The listing builds one solid part. Answer for the finished solid, in the listing's coordinates (mm). A direction names the side the tool comes from. Give positions to 0.01 mm unless a question says otherwise; leave off trailing zeros. Write each loop counter-clockwise with the first axis right and the second up, starting at its lowest first coordinate (ties: lowest second). Pieces come first, ordered by that corner, then holes. Notation, with made-up numbers: (24.5, 85) -> (32.5, 85) arc R30 ccw to (32.5, 119) -> close; hole circle Ø11 at (49, 0). An arc over 180 degrees is marked (long way). Put each result on its own line as item: value. Start each with the question number.
1) A cutting plane is placed at C-C (y = -26.5). Write down the section's boundary in (x, z), then the cut area to 3 significant figures.
2) Flat-ended cylindrical pins translate along their axes: pin 1 Ø1 at (y, z) = (-30, -13.5) entering from -X; pin 2 Ø8 at (x, y) = (2.5, -33.5) entering from -Z; pin 3 Ø1.5 at (x, y) = (16.5, -15.5) entering from -Z; pin 4 Ø5.5 at (x, z) = (0, 0) entering from -Y. Find the tip coordinate at first contact, or state that the pin passes through.
3) For a pull along X with two mould halves and no side action, classify faces 1 (the conical face through (31.82, -14.81, -7.07)), 2 (the flat face through (-17, -2, -14)), 3 (the flat face through (0, 0, -6)) as released by +X, released by -X, zero draft, split by the parting line, or undercut.
4) A cutting plane is placed at B-B (y = -8). Give the number of separate pieces and of enclosed holes in the cut face, then the cut area to 3 significant figures.
5) Find the intervals of material crossed by line 1 along X through (y, z) = (-6, 0); line 2 along X through (y, z) = (-3.5, 0); line 3 along X through (y, z) = (-41, -33.5), in increasing order. Write a range as from..to.
6) For faces 4 (the cylindrical face through (14.087, -52.986, -44.734)), 5 (the flat face through (14, -2, 17)), 6 (the cylindrical face through (9.36, -11.52, -5.97)), determine the directions among +Z, -Z, +X, -X, +Y, -Y from which every point of the face is accessible in a straight line to the end or side of a thin tool.
7) A cutting plane is placed at A-A (y = -34). Write down the section's boundary in (x, z), then the cut area to 3 significant figures.
from build123d import *

# Parameters (mm, degrees)
SKETCH_2_R          = 1.75
CUT_EXTRUDE_1_DEPTH = 85.280602751
CUT_EXTRUDE_2_DEPTH = 8
SKETCH_4_R          = 3
CUT_EXTRUDE_3_DEPTH = 2
SKETCH_5_R          = 11.1
CUT_EXTRUDE_4_DEPTH = 2.2
SKETCH_6_R          = 4.5
CUT_EXTRUDE_5_DEPTH = 79.292911557
SKETCH_7_R          = 46.9
SKETCH_7_R_2        = 40
EXTRUDE_1_DEPTH     = 2


with BuildPart() as part:
    # 草图1 → 旋转1 (revolve)
    with BuildSketch(Plane.XY, mode=Mode.PRIVATE) as revolve_1_sk:
        Polygon((0, 0), (26.9, 0), (46.9, -52), (43.553846154, -52), (28.4, -12.6), (26.9, -12.6), (0, -12.6), align=None)
    revolve(revolve_1_sk.sketch.rotate(Axis((0, 0, 0), (0, -1, 0)), 90), axis=Axis((0, 0, 0), (0, -1, 0)))

    # 草图2 → 切除-拉伸1 (cut, through all)
    with BuildSketch(Plane(origin=(0, 0, 0), x_dir=(1, 0, 0), z_dir=(0, 1, 0))):
        with BuildLine():
            Line((-15.5, 13.75), (-15.5, 15.5))
            Line((-15.5, 15.5), (-13.75, 15.5))
            ThreePointArc((-13.75, 15.5), (-16.737436867, 16.737436867), (-15.5, 13.75))
        make_face()
        with BuildLine():
            Line((-13.75, 15.5), (-15.5, 15.5))
            Line((-15.5, 15.5), (-15.5, 13.75))
            ThreePointArc((-15.5, 13.75), (-14.262563133, 14.262563133), (-13.75, 15.5))
        make_face()
        with BuildLine():
            Line((-15.5, 13.75), (-15.5, 15.5))
            Line((-15.5, 15.5), (-13.75, 15.5))
            ThreePointArc((-13.75, 15.5), (-16.737436867, 16.737436867), (-15.5, 13.75))
        make_face()
        with BuildLine():
            Line((-13.75, 15.5), (-15.5, 15.5))
            Line((-15.5, 15.5), (-15.5, 13.75))
            ThreePointArc((-15.5, 13.75), (-14.262563133, 14.262563133), (-13.75, 15.5))
        make_face()
        with BuildLine():
            ThreePointArc((17.25, 15.5), (15.5, 17.25), (13.75, 15.5))
            Line((13.75, 15.5), (15.5, 15.5))
            Line((15.5, 15.5), (15.5, 13.75))
            ThreePointArc((15.5, 13.75), (16.737436867, 14.262563133), (17.25, 15.5))
        make_face()
        with BuildLine():
            Line((15.5, 15.5), (13.75, 15.5))
            ThreePointArc((13.75, 15.5), (14.262563133, 14.262563133), (15.5, 13.75))
            Line((15.5, 13.75), (15.5, 15.5))
        make_face()
        with BuildLine():
            ThreePointArc((17.25, 15.5), (15.5, 17.25), (13.75, 15.5))
            Line((13.75, 15.5), (15.5, 15.5))
            Line((15.5, 15.5), (15.5, 13.75))
            ThreePointArc((15.5, 13.75), (16.737436867, 14.262563133), (17.25, 15.5))
        make_face()
        with BuildLine():
            Line((15.5, 15.5), (13.75, 15.5))
            ThreePointArc((13.75, 15.5), (14.262563133, 14.262563133), (15.5, 13.75))
            Line((15.5, 13.75), (15.5, 15.5))
        make_face()
        with BuildLine():
            ThreePointArc((17.25, -15.5), (16.737436867, -14.262563133), (15.5, -13.75))
            Line((15.5, -13.75), (15.5, -15.5))
            Line((15.5, -15.5), (13.75, -15.5))
            ThreePointArc((13.75, -15.5), (15.5, -17.25), (17.25, -15.5))
        make_face()
        with BuildLine():
            Line((15.5, -15.5), (15.5, -13.75))
            ThreePointArc((15.5, -13.75), (14.262563133, -14.262563133), (13.75, -15.5))
            Line((13.75, -15.5), (15.5, -15.5))
        make_face()
        with BuildLine():
            ThreePointArc((17.25, -15.5), (16.737436867, -14.262563133), (15.5, -13.75))
            Line((15.5, -13.75), (15.5, -15.5))
            Line((15.5, -15.5), (13.75, -15.5))
            ThreePointArc((13.75, -15.5), (15.5, -17.25), (17.25, -15.5))
        make_face()
        with BuildLine():
            Line((15.5, -15.5), (15.5, -13.75))
            ThreePointArc((15.5, -13.75), (14.262563133, -14.262563133), (13.75, -15.5))
            Line((13.75, -15.5), (15.5, -15.5))
        make_face()
        with BuildLine():
            ThreePointArc((-13.75, -15.5), (-14.262563133, -14.262563133), (-15.5, -13.75))
            Line((-15.5, -13.75), (-15.5, -15.5))
            Line((-15.5, -15.5), (-13.75, -15.5))
        make_face()
        with BuildLine():
            Line((-15.5, -15.5), (-15.5, -13.75))
            ThreePointArc((-15.5, -13.75), (-16.737436867, -16.737436867), (-13.75, -15.5))
            Line((-13.75, -15.5), (-15.5, -15.5))
        make_face()
        with BuildLine():
            ThreePointArc((-13.75, -15.5), (-14.262563133, -14.262563133), (-15.5, -13.75))
            Line((-15.5, -13.75), (-15.5, -15.5))
            Line((-15.5, -15.5), (-13.75, -15.5))
        make_face()
        with BuildLine():
            Line((-15.5, -15.5), (-15.5, -13.75))
            ThreePointArc((-15.5, -13.75), (-16.737436867, -16.737436867), (-13.75, -15.5))
            Line((-13.75, -15.5), (-15.5, -15.5))
        make_face()
        with Locations(Location((0, 21.920310217, 0), (0, 0, 270))):
            Circle(SKETCH_2_R)
        with Locations(Location((-21.920310217, 0, 0), (0, 0, 270))):
            Circle(SKETCH_2_R)
        with Locations(Location((21.920310217, 0, 0), (0, 0, 270))):
            Circle(SKETCH_2_R)
        with Locations(Location((0, -21.920310217, 0), (0, 0, 270))):
            Circle(SKETCH_2_R)
    extrude(amount=-CUT_EXTRUDE_1_DEPTH, mode=Mode.SUBTRACT)

    # 草图3 → 切除-拉伸2 (cut)
    with BuildSketch(Plane.XZ.offset(12.6)):
        Polygon((2.086344802, -19.833965415), (0, -21.920310217), (-2.086344802, -19.833965415), (-3.290896534, -21.920310217), (-1.645448267, -24.770310217), (1.645448267, -24.770310217), (3.290896534, -21.920310217), align=None)
        Polygon((-2.086344802, -19.833965415), (0, -21.920310217), (2.086344802, -19.833965415), (1.645448267, -19.070310217), (-1.645448267, -19.070310217), align=None)
        Polygon((21.920310217, 0), (19.833965415, -2.086344802), (21.920310217, -3.290896534), (24.770310217, -1.645448267), (24.770310217, 1.645448267), (21.920310217, 3.290896534), (19.833965415, 2.086344802), align=None)
        Polygon((19.070310217, -1.645448267), (19.833965415, -2.086344802), (21.920310217, 0), (19.833965415, 2.086344802), (19.070310217, 1.645448267), align=None)
        Polygon((-3.290896534, 21.920310217), (-2.086344802, 19.833965415), (0, 21.920310217), (2.086344802, 19.833965415), (3.290896534, 21.920310217), (1.645448267, 24.770310217), (-1.645448267, 24.770310217), align=None)
        Polygon((0, 21.920310217), (-2.086344802, 19.833965415), (-1.645448267, 19.070310217), (1.645448267, 19.070310217), (2.086344802, 19.833965415), align=None)
        Polygon((-21.920310217, -3.290896534), (-19.833965415, -2.086344802), (-21.920310217, 0), (-19.833965415, 2.086344802), (-21.920310217, 3.290896534), (-24.770310217, 1.645448267), (-24.770310217, -1.645448267), align=None)
        Polygon((-21.920310217, 0), (-19.833965415, -2.086344802), (-19.070310217, -1.645448267), (-19.070310217, 1.645448267), (-19.833965415, 2.086344802), align=None)
    extrude(amount=-CUT_EXTRUDE_2_DEPTH, mode=Mode.SUBTRACT)

    # 草图4 → 切除-拉伸3 (cut)
    with BuildSketch(Plane(origin=(0, 0, 0), x_dir=(1, 0, 0), z_dir=(0, 1, 0))):
        with Locations(Location((-15.5, -15.5, 0), (0, 0, 270))):
            Circle(SKETCH_4_R)
        with Locations(Location((-15.5, 15.5, 0), (0, 0, 270))):
            Circle(SKETCH_4_R)
        with Locations(Location((15.5, 15.5, 0), (0, 0, 270))):
            Circle(SKETCH_4_R)
        with Locations(Location((15.5, -15.5, 0), (0, 0, 270))):
            Circle(SKETCH_4_R)
    extrude(amount=-CUT_EXTRUDE_3_DEPTH, mode=Mode.SUBTRACT)

    # 草图5 → 切除-拉伸4 (cut)
    with BuildSketch(Plane.XZ.offset(12.6)):
        with Locations(Location((0, 0, 0), (0, 0, 270))):
            Circle(SKETCH_5_R)
    extrude(amount=-CUT_EXTRUDE_4_DEPTH, mode=Mode.SUBTRACT)

    # 草图6 → 切除-拉伸5 (cut, through all)
    with BuildSketch(Plane.XZ.offset(10.4)):
        with Locations(Location((0, 0, 0), (0, 0, 270))):
            Circle(SKETCH_6_R)
    extrude(amount=-CUT_EXTRUDE_5_DEPTH, mode=Mode.SUBTRACT)

    # 草图7 → 凸台-拉伸1 (add)
    with BuildSketch(Plane.XZ.offset(52)):
        with Locations(Location((0, 0, 0), (0, 0, 270))):
            Circle(SKETCH_7_R)
        with Locations(Location((0, 0, 0), (0, 0, 270))):
            Circle(SKETCH_7_R_2, mode=Mode.SUBTRACT)
    extrude(amount=EXTRUDE_1_DEPTH)

    # 圆角1: read off the stored shape, not the designer's step
    # 圆角1 outline → 圆角1 (revolve)
    with BuildSketch(Plane.XY):
        with BuildLine():
            Line((43.553846154, -43.866224222), (40.425470855, -43.866224222))
            ThreePointArc((40.425470855, -43.866224222), (41.078361572, -47.978392274), (40, -52))
            Line((40, -52), (43.553846154, -52))
            Line((43.553846154, -52), (43.553846154, -43.866224222))
        make_face()
    revolve(axis=Axis((0, 0, 0), (0, 1, 0)))


solid = part.part
Reply:
1. outline: circle Ø74.18 at (0, 0); hole circle Ø67.49 at (0, 0)
1. area: 745 mm2
2. pin 1: stops at x = -36.27
2. pin 2: stops at z = -41.26
2. pin 3: stops at z = -28.96
2. pin 4: passes through
3. face 1: split by the parting line
3. face 2: undercut
3. face 3: zero draft
4. separate pieces: 1
4. enclosed holes: 9
4. area: 2,610 mm2
5. line 1: x = -29.21..-24.77, -19.07..-4.5, 4.5..19.07, 24.77..29.21
5. line 2: x = -28.25..-23.67, -20.17..-4.5, 4.5..20.17, 23.67..28.25
5. line 3: x = -26.43..-20.59, 20.59..26.43
6. face 4: +Y, -Y
6. face 5: +Y
6. face 6: -Y
7. outline: circle Ø79.95 at (0, 0); hole circle Ø73.26 at (0, 0)
7. area: 805 mm2
